from build123d import *

# Parameters (mm, degrees)
BOSS_EXTRUDE1_DEPTH      = 10
BOSS_EXTRUDE1_DEPTH_BACK = 10
BOSS_EXTRUDE2_DEPTH      = 10
SKETCH3_W                = 150
SKETCH3_H                = 20
BOSS_EXTRUDE3_DEPTH      = 10


with BuildPart() as part:
    # Sketch1 → Boss-Extrude1 (new, two sides: drawn at the far end of the back side and taken through both)
    with BuildSketch(Plane.XY.offset(-BOSS_EXTRUDE1_DEPTH_BACK)):
        Polygon((0, 0), (150, 0), (14.053831945, 63.392739261), align=None)
    extrude(amount=BOSS_EXTRUDE1_DEPTH + BOSS_EXTRUDE1_DEPTH_BACK)



with BuildPart() as body_2:
    # Sketch2 → Boss-Extrude2 (new body)
    with BuildSketch(Plane(origin=(26.790929274, 57.453333234, 0), x_dir=(0.9063077870366495, -0.42261826174070033, 0), z_dir=(0.42261826174070033, 0.9063077870366495, 0))):
        Polygon((68.803496006, 65.613486746), (-21.196503994, 65.613486746), (-21.196503994, -64.386513254), (68.803496006, -64.386513254), (135.946168055, -39.948579179), (135.946168055, -10), (-14.053831945, -10), (-14.053831945, 10), (135.946168055, 10), (135.946168055, 41.175552671), align=None)
    extrude(amount=BOSS_EXTRUDE2_DEPTH)


with BuildPart() as part_1:
    add(part.part)

    add(body_2.part)  # Boss-Extrude3 merges body 2
    # Sketch3 → Boss-Extrude3 (add)
    with BuildSketch(Plane(origin=(26.790929274, 57.453333234, 0), x_dir=(0.9063077870366495, -0.42261826174070033, 0), z_dir=(0.42261826174070033, 0.9063077870366495, 0))):
        with Locations((60.946168055, 0)):
            Rectangle(SKETCH3_W, SKETCH3_H)
    extrude(amount=BOSS_EXTRUDE3_DEPTH)


solid = part_1.part
Geometry: final body of the model. Coordinates: model frame, mm. A direction names the side the tool comes from. Give positions to 0.01 mm unless a question says otherwise; leave off trailing zeros. Write each loop counter-clockwise with the first axis right and the second up, starting at its lowest first coordinate (ties: lowest second). Pieces come first, ordered by that corner, then holes.
(1) Cut plane C-C, the plane z = -4. Return loops of the section in (x, y), then the cut area to 3 significant figures.
(2) Cut plane A-A, the plane x = 20. Return loops of the section in (y, z), then the cut area to 3 significant figures.
(3) Mould query, pull axis Y, two halves, no side actions, for faces 3 (the flat face through (57, 18, -10)), 4 (the flat face through (7.125, 32.14, -0.14)), 5 (the flat face through (152.1, 4.5, 0)). Classes: released by +Y, released by -Y, zero draft, split by the parting line, or undercut.
(4) Cut plane B-B, the plane y = 31. Return loops of the section in (x, z), then the cut area to 3 significant figures.
(5) Ray query, line 1 (Z direction, x = 94.5, y = 21); line 2 (Y direction, x = 145.5, z = -26); line 3 (Y direction, x = 57, z = 36.5). Return the intervals inside material, ascending.
(6) First-contact query: P1, Ø3, axis at x = 117, z = -35, coming from the -Y side; P2, Ø12, axis at x = 45.5, z = -41, coming from the +Y side; P3, Ø12, axis at x = 109.5, y = 32.5, coming from the -Z side. Flat tips, straight axial feed; report the tip coordinate or a pass-through.
(7) Cut plane D-D, the plane x = 35.5. Return loops of the section in (y, z).
(8) Access query for faces 1 (the flat face through (57, 18, 10)), 2 (the flat face through (9.664, 70.879, -1.523)). Directions: +Z, -Z, +X, -X, +Y, -Y. A direction counts if a zero-diameter tool reaches every point of the face in a straight line with its end or side. Return the directions, or none.
Values follow:
1. outline: (0, 0) - (150, 0) - (154.23, 9.06) - (11.81, 75.47) - (7.58, 66.41) - (14.05, 63.39) - close
1. area: 6,330 mm2
2. outline: (0, -10) - (60.62, -10) - (60.62, -65.61) - (71.65, -65.61) - (71.65, 64.39) - (60.62, 64.39) - (60.62, 10) - (0, 10) - close
2. area: 2,650 mm2
3. face 3: zero draft
3. face 4: undercut
3. face 5: released by -Y
4. outline: (6.87, -10) - (83.52, -10) - (83.52, -65.61) - (90.37, -65.61) - (107.18, -60.07) - (107.18, 58.84) - (90.37, 64.39) - (83.52, 64.39) - (83.52, 10) - (6.87, 10) - close
4. area: 4,520 mm2
5. line 1: z = -10 to 10
5. line 2: y = 2.1 to 13.13
5. line 3: y = 43.37 to 54.4
6. P1: stops at y = 14.69
6. P2: stops at y = 62.56
6. P3: stops at z = -61.55
7. outline: (0, -10) - (53.39, -10) - (53.39, -65.61) - (64.43, -65.61) - (64.43, 64.39) - (53.39, 64.39) - (53.39, 10) - (0, 10) - close
8. face 1: +Z, -X, -Y
8. face 2: +Z, -Z, -X, +Y
